Could you check a few things on this model? Use its own coordinates, in mm. Round coordinates to 2 decimals unless told otherwise and drop trailing zeros. Write each loop counter-clockwise with the first axis right and the second up, starting at its lowest first coordinate (ties: lowest second). Pieces come first, ordered by that corner, then holes.
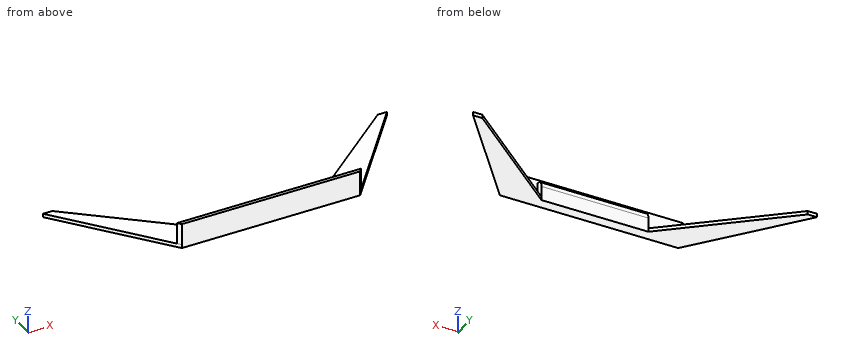
```python
from build123d import *

# Parameters (mm, degrees)
F1_DEPTH    = 1
F3_DEPTH    = 6
F2_W        = 30
F2_H        = 2
F4_DEPTH    = 5
F5_T1_DEPTH = 40


# Not quite as in the source:
# - a fillet or chamfer that OpenCascade refuses, or shapes differently, is made with other operations: its cross-section is extruded or revolved along the edge and cut away or added


with BuildPart() as f1:
    # F0 (on Top) → F1 (new body)
    with BuildSketch(Plane.XY):
        Polygon((15, 0), (0, 0), (-15, 0), (-45.6417777248, 25.7115043875), (-48.2388163507, 25.7115043875), (-25, -3), (0, -3), (25, -3), (48.2388163507, 25.7115043875), (45.6417777248, 25.7115043875), align=None)
    extrude(amount=F1_DEPTH)

    # F2 (on face) → F3 (join)
    with BuildSketch(Plane.XY.offset(1)):
        Polygon((-15, -2), (-25.8093904115, -2), (-25, -3), (25, -3), (25.8093904115, -2), (15, -2), align=None)
    extrude(amount=F3_DEPTH)

    # F2 (on face) → F4 (join)
    with BuildSketch(Plane.XY.offset(1)):
        with Locations((0, -1)):
            Rectangle(F2_W, F2_H)
    extrude(amount=F4_DEPTH)

    # F5: fillet of radius 2 on 1 edges, made by hand

    # F5_s2 → F5_t1 (cut)
    with BuildSketch(Plane.YZ.offset(-20)):
        with BuildLine():
            add(Edge.make_bspline(
                [(0, 4), (0, 6), (-2, 6)],
                knots=[0, 0, 0, 1, 1, 1], degree=2, weights=[1, 1, 1]))
            Line((-2, 6), (0, 6))
            Line((0, 6), (0, 4))
        make_face()
    extrude(amount=F5_T1_DEPTH, mode=Mode.SUBTRACT)


solid = f1.part
```
Q1. Imagine slicing it at C-C, the plane x = -22.5. Write out the boundary of the cut face in (y, z).
Q2. I'm going to push flat-ended pins straight in: pin 1 Ø3 at (x, z) = (10, 3) entering from +Y; pin 2 Ø1.6 at (y, z) = (-1.5, 4.5) entering from +X; pin 3 Ø2 at (y, z) = (0.5, 1.5) entering from -X. Where does each tip first touch, or does it pass through?
Q3. If I drill on L1, parallel to X at y = -0.25, z = 2.5; L2, parallel to Y at x = -7, z = 1; L3, parallel to Z at x = 27, y = 2, over which ranges is the centre line in solid material (lowest first)?
Q4. Imagine slicing it at A-A, the plane z = 3. Write out the boundary of the cut face in (x, y).
Q5. Imagine slicing it at B-B, the plane y = 11. Write out the boundary of the cut face in (x, z).
Q6. Imagine slicing it at D-D, the plane y = 4. Write out the boundary of the cut face in (x, z), then the cut area to 3 significant figures.
Results found:
1. outline: (-3, 0) - (6.29, 0) - (6.29, 1) - (-2, 1) - (-2, 7) - (-3, 7) - close
2. pin 1: stops at y = 0
2. pin 2: stops at x = 25.81
2. pin 3: stops at x = -28.53
3. L1: x = -15 to 15
3. L2: y = -3 to 0
3. L3: z = 0 to 1
4. outline: (-25.81, -2) - (-25, -3) - (25, -3) - (25.81, -2) - (15, -2) - (15, 0) - (-15, 0) - (-15, -2) - close
5. outline: (-36.33, 0) - (-28.11, 0) - (-28.11, 1) - (-36.33, 1) - close; (28.11, 0) - (36.33, 0) - (36.33, 1) - (28.11, 1) - close
6. outline: (-30.67, 0) - (-19.77, 0) - (-19.77, 1) - (-30.67, 1) - close; (19.77, 0) - (30.67, 0) - (30.67, 1) - (19.77, 1) - close
6. area: 21.8 mm2
